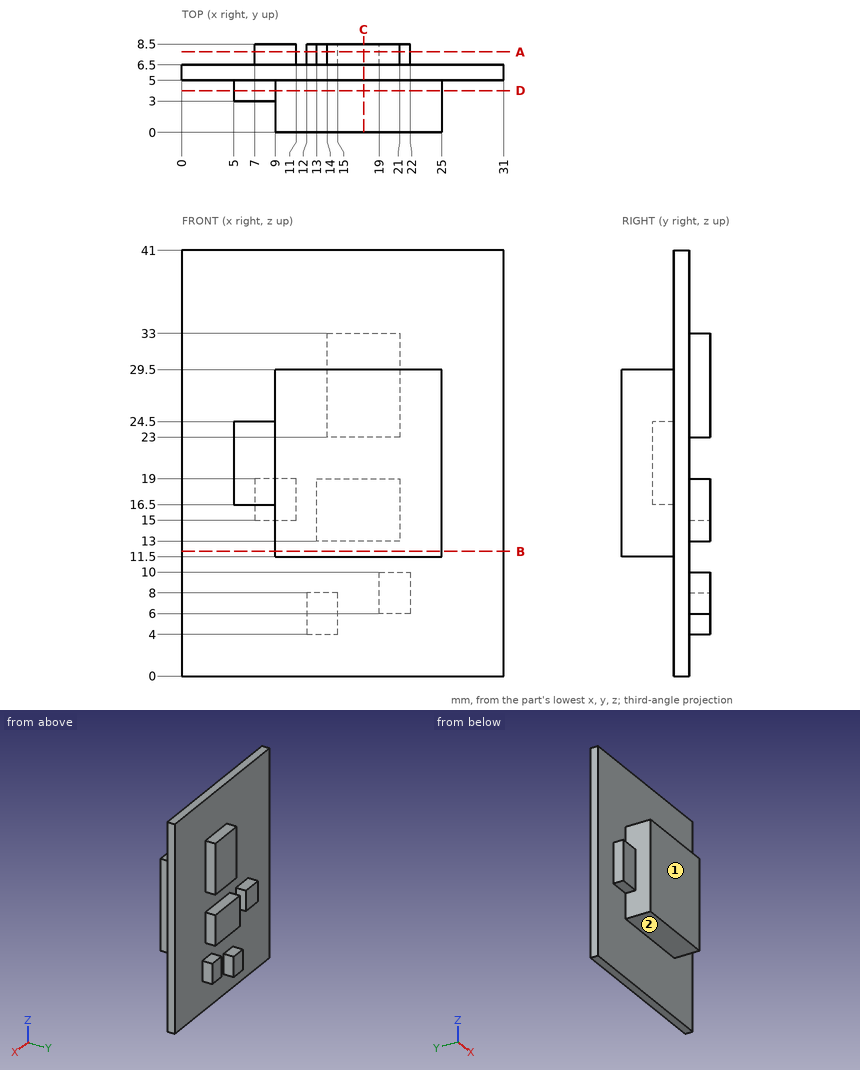
Can you work these out from the drawing? Everything is in mm from the part's minimum corner. A direction names the side the tool comes from. Give positions to 0.01 mm unless a question says otherwise; leave off trailing zeros. Loops run counter-clockwise (first coordinate to the right, second up) from the corner with the lowest first, then second, coordinate; pieces in that order, holes last. Notation, with made-up numbers: (87, 81.25) -> (139, 81.25) arc R16 cw to (139, 99.25) -> close; hole circle Ø5 at (75, 70). An arc over 180 degrees is marked (long way). Return JSON: item names as keys, results as strings.
Item 1: I'm going to push flat-ended pins straight in: pin 1 (1.5 mm diameter, centred on x = 17, y = 3.5, fed in from +Z); pin 2 (1 mm diameter, centred on y = 7.5, z = 17.5, fed in from -X); pin 3 (0.6 mm diameter, centred on y = 7.5, z = 8, fed in from -X). Where does each tip first touch, or does it pass through?
Geometry results:
{"pin 1": "stops at z = 29.5", "pin 2": "stops at x = 7", "pin 3": "stops at x = 12"}
Item 2: If we section it at A-A on y = 7.75: List the corners of the cut face in (x, z) for me, plus the area to 3 significant figures.
Geometry results:
{"outline": "(7, 15) -> (11, 15) -> (11, 19) -> (7, 19) -> close; (12, 4) -> (15, 4) -> (15, 8) -> (12, 8) -> close; (13, 13) -> (21, 13) -> (21, 19) -> (13, 19) -> close; (14, 23) -> (21, 23) -> (21, 33) -> (14, 33) -> close; (19, 6) -> (22, 6) -> (22, 10) -> (19, 10) -> close", "area": "158 mm²"}
Item 3: If we section it at D-D on y = 4: List the corners of the cut face in (x, z) for me.
Geometry results:
{"outline": "(5, 16.5) -> (9, 16.5) -> (9, 11.5) -> (25, 11.5) -> (25, 29.5) -> (9, 29.5) -> (9, 24.5) -> (5, 24.5) -> close"}
Item 4: If we section it at B-B on z = 12: List the corners of the cut face in (x, y) for me, plus the area to 4 significant figures.
Geometry results:
{"outline": "(0, 5) -> (9, 5) -> (9, 0) -> (25, 0) -> (25, 5) -> (31, 5) -> (31, 6.5) -> (0, 6.5) -> close", "area": "126.5 mm²"}
Item 5: I need wall thicknesses on L1, parallel to X at y = 6.75, z = 5.5; L2, parallel to Y at x = 23, z = 8.5; L3, parallel to X at y = 1.75, z = 12.5. Which ranges of each line are inside material? Lowest first, please. Write a range as from..to.
Geometry results:
{"L1": "x = 12..15", "L2": "y = 5..6.5", "L3": "x = 9..25"}
Item 6: If we section it at C-C on x = 17.5: List the corners of the cut face in (y, z) for me, plus the area to 4 significant figures.
Geometry results:
{"outline": "(0, 11.5) -> (5, 11.5) -> (5, 0) -> (6.5, 0) -> (6.5, 13) -> (8.5, 13) -> (8.5, 19) -> (6.5, 19) -> (6.5, 23) -> (8.5, 23) -> (8.5, 33) -> (6.5, 33) -> (6.5, 41) -> (5, 41) -> (5, 29.5) -> (0, 29.5) -> close", "area": "183.5 mm²"}
Item 7: Which directions (+Z, -Z, +X, -X, +Y, -Y) give clear straight access to the entire face, cutting with the end or side of a thin tool? Please do the marked faces 1 and 2.
Geometry results:
{"face 1": "+Z, -Z, +X, -X, -Y", "face 2": "-Z, +X, -X, -Y"}
